Could you check a few things on this model? Use its own coordinates, in mm. A direction names the side the tool comes from. Coordinates: 2 decimals unless noted, no trailing zeros. Order: outer loops, then holes, each group sorted by start corner. A loop starts at its lowest first (then second) coordinate and runs counter-clockwise, first axis right, second up. Notation, with made-up numbers: (48.5, 61) - (91.5, 61) arc R15 cw to (91.5, 68) - close; hole circle Ø1 at (84, 49.25). An arc over 180 degrees is marked (long way). Answer as CSV lines item,"result". Start each with the question number.
1. For faces 4 (the face through (-2, 77, 152.4)), 5 (the face through (50.8, 75, 75)), which set-ups out of +Z, -Z, +X, -X, +Y, -Y let a thin tool reach every point of the face, with its end or its side?
2. I need wall thicknesses on probe 1 along Z at (x, y) = (33.5, 45.5); probe 2 along X at (y, z) = (36.5, 46). Which ranges of each line are inside material? Lowest first, please.
3. Thinking about a two-plate mould opening in Z: for faces 1 (the face through (-2, 77, 0)), 2 (the face through (-50.8, 75, 77)), 3 (the face through (74.78, 75, 75)), which applies, released by +Z, released by -Z, zero draft, split by the parting line, or undercut?
4. I want a section at C-C, the plane x = -16. List the corners of the cut face in (y, z) for me.
5. I want a section at B-B, the plane y = 10. List the corners of the cut face in (x, z) for me, and give its area (3 significant figures).
6. For pin 1 (5 mm diameter, centred on x = 3.5, y = 62.5, fed in from -Z), with a flat end and sliding along its axis, tell me the tip position at first contact or that it passes through.
7. I want a section at A-A, the plane z = 73. List the corners of the cut face in (x, y) for me.
from build123d import *

# Parameters (mm, degrees)
F0_W     = 152.4
F0_H     = 152.4
F1_DEPTH = 152.4
F2_W     = 50.8
F2_H     = 50.8
F3_DEPTH = 152.4


with BuildPart() as f1:
    # F0 (on Top) → F1 (new body)
    with BuildSketch(Plane.XY):
        with Locations((-1.420007, 76.2)):
            Rectangle(F0_W, F0_H)
    extrude(amount=F1_DEPTH)

    # F2 (on face) → F3 (cut)
    with BuildSketch(Plane.XZ):
        with Locations((-25.4, 101.6)):
            Rectangle(F2_W, F2_H)
        with Locations((25.4, 101.6)):
            Rectangle(F2_W, F2_H)
        with Locations((25.4, 50.8)):
            Rectangle(F2_W, F2_H)
        with Locations((-25.4, 50.8)):
            Rectangle(F2_W, F2_H)
    extrude(amount=-F3_DEPTH, mode=Mode.SUBTRACT)


solid = f1.part
Solved:
1,face 4,"+Z, +X, -X, +Y, -Y"
1,face 5,"+Y, -Y"
2,probe 1,"z = 0 to 25.4, 127 to 152.4"
2,probe 2,"x = -77.62 to -50.8, 50.8 to 74.78"
3,face 1,"released by -Z"
3,face 2,"undercut"
3,face 3,"zero draft"
4,outline,"(0, 0) - (152.4, 0) - (152.4, 25.4) - (0, 25.4) - close; (0, 127) - (152.4, 127) - (152.4, 152.4) - (0, 152.4) - close"
5,outline,"(-77.62, 0) - (74.78, 0) - (74.78, 152.4) - (-77.62, 152.4) - close; hole (-50.8, 25.4) - (50.8, 25.4) - (50.8, 127) - (-50.8, 127) - close"
5,area,"12,900 mm2"
6,pin 1,"stops at z = 0"
7,outline,"(-77.62, 0) - (-50.8, 0) - (-50.8, 152.4) - (-77.62, 152.4) - close; (50.8, 0) - (74.78, 0) - (74.78, 152.4) - (50.8, 152.4) - close"
